```python
from build123d import *

# Parameters (mm, degrees)
SKETCH1_R               = 37.5
SKETCH1_R_2             = 27.5
BOSS_EXTRUDE1_DEPTH     = 5
BOSS_EXTRUDE2_DEPTH     = 10
SKETCH3_R               = 27.5
CUT_EXTRUDE2_DEPTH      = 6
CUT_EXTRUDE3_DEPTH      = 58.034295486
CUT_EXTRUDE3_DEPTH_BACK = 58.034295486
SKETCH4_R               = 3
SKETCH5_R               = 1.5
CUT_EXTRUDE4_DEPTH      = 56.927728914


with BuildPart() as part:
    # Sketch1 → Boss-Extrude1 (new body)
    with BuildSketch(Plane(origin=(0, 0, 0), x_dir=(1, 0, 0), z_dir=(0, 1, 0))):
        with Locations(Location((0, 0, 0), (0, 0, 270))):
            Circle(SKETCH1_R)
        with Locations(Location((0, 0, 0), (0, 0, 270))):
            Circle(SKETCH1_R_2, mode=Mode.SUBTRACT)
    extrude(amount=BOSS_EXTRUDE1_DEPTH)

    # Sketch2 → Boss-Extrude2 (add)
    with BuildSketch(Plane(origin=(0, 5, 0), x_dir=(1, 0, 0), z_dir=(0, 1, 0))):
        with BuildLine():
            Line((0, 31), (-40.269850528, 31))
            Line((-40.269850528, 31), (-40.269850528, -31))
            Line((-40.269850528, -31), (0, -31))
            ThreePointArc((0, -31), (31, 0), (0, 31))
        make_face()
    extrude(amount=BOSS_EXTRUDE2_DEPTH)

    # Sketch3 → Cut-Extrude2 (cut)
    with BuildSketch(Plane.XZ.offset(-5)):
        with Locations(Location((0, 0, 0), (0, 0, 90))):
            Circle(SKETCH3_R)
    extrude(amount=-CUT_EXTRUDE2_DEPTH, mode=Mode.SUBTRACT)

    # Sketch4 → Cut-Extrude3 (cut, two sides: drawn at the far end of the back side and taken through both)
    with BuildSketch(Plane(origin=(0, 15, 0), x_dir=(1, 0, 0), z_dir=(0, 1, 0)).offset(-CUT_EXTRUDE3_DEPTH_BACK)):
        with Locations(Location((0, 0, 0), (0, 0, 270))):
            Circle(SKETCH4_R)
    extrude(amount=CUT_EXTRUDE3_DEPTH + CUT_EXTRUDE3_DEPTH_BACK, mode=Mode.SUBTRACT)

    # Sketch5 → Cut-Extrude4 (cut, through all)
    with BuildSketch(Plane(origin=(0, 5, 0), x_dir=(1, 0, 0), z_dir=(0, 1, 0))):
        with Locations(Location((34.5, 0, 0), (0, 0, 270))):
            Circle(SKETCH5_R)
        with Locations(Location((0, -34.5, 0), (0, 0, 270))):
            Circle(SKETCH5_R)
        with Locations(Location((-34.5, 0, 0), (0, 0, 270))):
            Circle(SKETCH5_R)
        with Locations(Location((0, 34.5, 0), (0, 0, 270))):
            Circle(SKETCH5_R)
    extrude(amount=-CUT_EXTRUDE4_DEPTH, mode=Mode.SUBTRACT)


solid = part.part
```
For this review, take the finished solid that the model builds, in its own axes (mm). A direction names the side the tool comes from. Round coordinates to 2 decimals unless told otherwise and drop trailing zeros. Order: outer loops, then holes, each group sorted by start corner. A loop starts at its lowest first (then second) coordinate and runs counter-clockwise, first axis right, second up. Notation, with made-up numbers: (89, 32.5) -> (107, 32.5) arc R23 cw to (107, 68.5) -> close; hole circle Ø1 at (62, 62). An arc over 180 degrees is marked (long way). Use a Markdown table: item, result.
Item 1: Take a section at C-C (y = 13.5). State the section outline as (x, z) points.
Resolved:
| item | result |
|---|---|
| outline | (-40.27, -31) -> (0, -31) arc R31 ccw to (0, 31) -> (-40.27, 31) -> close; hole circle Ø6 at (0, 0) |
Item 2: For line 1 along X through (y, z) = (1.2, 0); line 2 along X through (y, z) = (2.5, -17.5); line 3 along X through (y, z) = (7, 1), list the stretches that pass through material, from the lowest coordinate up. Write a range as [from, to].
Resolved:
| item | result |
|---|---|
| line 1 | x = [-37.5, -36], [-33, -27.5], [27.5, 33], [36, 37.5] |
| line 2 | x = [-33.17, -21.21], [21.21, 33.17] |
| line 3 | x = [-40.27, -27.48], [27.48, 30.98] |
Item 3: Machinability: for faces 4 (the flat face through (-20, 10, 31)), 5 (the flat face through (32, 5, 0)), 6 (the cylindrical face through (-24.397, 5.423, 12.69)), 7 (the flat face through (-20, 10, -31)), which of the approach directions +Z, -Z, +X, -X, +Y, -Y give a long, thin tool a straight path to every point of the face, cutting with its end or side? Answer none if there is none.
Resolved:
| item | result |
|---|---|
| face 4 | +Z, +X, -X, +Y |
| face 5 | +X, +Y |
| face 6 | -Y |
| face 7 | -Z, +X, -X, +Y |
Item 4: Take a section at B-B (z = 34.5). State the section outline as (x, y) points, plus the area to 3 significant figures.
Resolved:
| item | result |
|---|---|
| outline | (-14.7, 0) -> (-1.5, 0) -> (-1.5, 5) -> (-14.7, 5) -> close; (1.5, 0) -> (14.7, 0) -> (14.7, 5) -> (1.5, 5) -> close |
| area | 132 mm² |
Item 5: Draft analysis for pull direction X (two halves, no side actions). For faces 1 (the cylindrical face through (-22.818, 2.465, -29.759)), 2 (the cylindrical face through (0.9, 12.97, 2.86)), 3 (the flat face through (-39, 5, 0)), state which applies: +X half, -X half, draft (parallel to the pull), parting line (faces both ways), or undercut.
Resolved:
| item | result |
|---|---|
| face 1 | parting line |
| face 2 | undercut |
| face 3 | draft |
Item 6: For pin 1 (4 mm diameter, centred on x = 0, z = 34.5, fed in from +Y); pin 2 (8 mm diameter, centred on x = 0, z = 0, fed in from -Y); pin 3 (5 mm diameter, centred on y = 10, z = 14.5, fed in from +X); pin 4 (1.5 mm diameter, centred on x = 14.5, z = -25.5, fed in from -Y), all flat-tipped, find the tip position at first contact; note any pin that passes through.
Resolved:
| item | result |
|---|---|
| pin 1 | stops at y = 5 |
| pin 2 | stops at y = 11 |
| pin 3 | stops at x = 28.58 |
| pin 4 | stops at y = 0 |
Item 7: Take a section at A-A (z = 0). State the section outline as (x, y) points, plus the area to 3 significant figures.
Resolved:
| item | result |
|---|---|
| outline | (-40.27, 5) -> (-37.5, 5) -> (-37.5, 0) -> (-36, 0) -> (-36, 5) -> (-33, 5) -> (-33, 0) -> (-27.5, 0) -> (-27.5, 11) -> (-3, 11) -> (-3, 15) -> (-40.27, 15) -> close; (3, 11) -> (27.5, 11) -> (27.5, 0) -> (33, 0) -> (33, 5) -> (31, 5) -> (31, 15) -> (3, 15) -> close; (36, 0) -> (37.5, 0) -> (37.5, 5) -> (36, 5) -> close |
| area | 429 mm² |
Item 8: Take a section at D-D (x = 15.5). State the section outline as (y, z) points.
Resolved:
| item | result |
|---|---|
| outline | (0, -34.15) -> (5, -34.15) -> (5, -26.85) -> (15, -26.85) -> (15, 26.85) -> (5, 26.85) -> (5, 34.15) -> (0, 34.15) -> (0, 22.72) -> (11, 22.72) -> (11, -22.72) -> (0, -22.72) -> close |
